Autodesk Inventor part; units mm, degrees
ref_plane "Arbeitsebene4" through (-9, 9, 0) normal (0, -0.8333, -0.5529) x (1, 0, 0)
ref_plane "YZ Plane" through (0, 0, 0) normal (1, 0, 0) x (0, 1, 0)
ref_plane "XZ Plane" through (0, 0, 0) normal (0, 1, 0) x (-1, 0, 0)
sketch "Skizze1" plane through (0, 0, 0) normal (0, 0, 1) x (1, 0, 0)
  line L0 (-12.6, 0) -> (12.6, 0) construction
  line L1 (0, -12.6) -> (0, 12.6) construction
  circle A0 centre (0, 0) radius 9
  circle A1 centre (0, 0) radius 8
  line L2 (-9, 9) -> (9, 9)
  dimension "d0" = 18
  dimension "d1" = 16
extrude "Extrusion4" add sketch "Skizze1" along normal blind 400 contours A0 | A1
extrude "Extrusion5" cut sketch "Skizze1" along normal through all contours A1
ref_plane "Arbeitsebene4" through (-9, 9, 0) normal (0, -0.8333, -0.5529) x (1, 0, 0)
split "Trennen5" plane through (-9, 9, 0) removes the side toward (0, -0.8333, -0.5529)
sketch "Skizze5" plane through (0, 0, 400) normal (0, 0, 1) x (1, 0, 0)
  circle A0 centre (0, 0) radius 8
  circle A1 centre (0, 0) radius 9
  dimension "d17" = 16
  dimension "d18" = 18
extrude "Extrusion6" add sketch "Skizze5" along normal blind 5
properties part number "Schräges Rohr CF16"
Geometry check sheet. Reference: the model listing, model coordinates, mm. Coordinates: 2 decimals unless noted, no trailing zeros. Loops run counter-clockwise (first coordinate to the right, second up) from the corner with the lowest first, then second, coordinate; pieces in that order, holes last. Notation, with made-up numbers: (-16.5, -39.5) -> (32.5, -39.5) arc R37 ccw to (32.5, -0.5) -> close; hole circle Ø1 at (35.25, 46). An arc over 180 degrees is marked (long way). Put each result on its own line as item: value.
1) Thickness scan on line 1 (Y direction, x = 0, z = 251); line 2 (Y direction, x = 1, z = 49.5). Record the ranges inside material, lowest first.
Result set:
line 1: y = -9 to -8, 8 to 9
line 2: y = -8.94 to -7.94, 7.94 to 8.94
2) Release check for a two-part mould opening along Y. For faces 1 (the flat face through (-8.042, 1.375, 11.491)), 2 (the cylindrical face through (-1.73, 7.81, 200.41)), 3 (the cylindrical face through (-1.951, 8.786, 199.664)) record: released by +Y, released by -Y, zero draft, split by the parting line, or undercut.
Result set:
face 1: released by -Y
face 2: undercut
face 3: split by the parting line
3) Gauge pin test, flat ends, axial feed: pin 1 Ø5 at (x, y) = (5, -1.5) entering from -Z; pin 2 Ø1 at (x, z) = (6.5, 116) entering from -Y; pin 3 Ø4 at (y, z) = (3, 50) entering from +X; pin 4 Ø1.5 at (y, z) = (-4.5, 120) entering from +X. Record the tip position at first contact, or that the pin passes through.
Result set:
pin 1: passes through
pin 2: stops at y = -6.71
pin 3: stops at x = 8.94
pin 4: stops at x = 8.18
4) Cross-section at C-C on z = 288. Record the boundary of the cut face in (x, y).
Result set:
outline: circle Ø18 at (0, 0); hole circle Ø16 at (0, 0)
5) Cross-section at A-A on x = 4.5. Record the boundary of the cut face in (y, z), plus the area to 3 significant figures.
Result set:
outline: (-7.79, 25.31) -> (-6.61, 23.53) -> (-6.61, 405) -> (-7.79, 405) -> close; (6.61, 3.6) -> (7.79, 1.82) -> (7.79, 405) -> (6.61, 405) -> close
area: 924 mm^2
6) Cross-section at B-B on y = 0. Record the boundary of the cut face in (x, z), plus the area to 3 significant figures.
Result set:
outline: (-9, 13.56) -> (-8, 13.56) -> (-8, 405) -> (-9, 405) -> close; (8, 13.56) -> (9, 13.56) -> (9, 405) -> (8, 405) -> close
area: 783 mm^2
